Check sheet for the drawn part. Datum: minimum x, y, z corner. Units: mm. A direction names the side the tool comes from. Round coordinates to 2 decimals unless told otherwise and drop trailing zeros. Put each result on its own line as item: value.
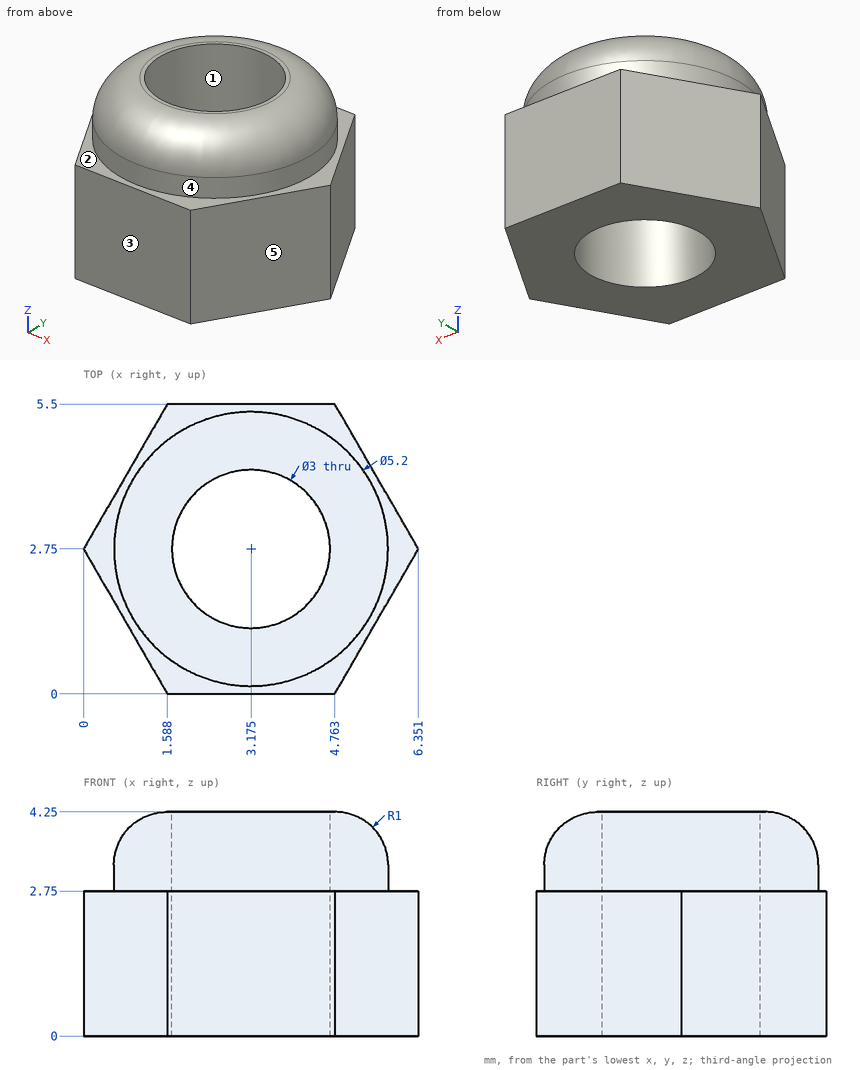
1. Access from +Z, -Z, +X, -X, +Y, -Y to the whole of each face (thin tool, end or side, straight path). Record for the marked faces 4 and 5.
Computed values:
face 4: +Z
face 5: +Z, -Z, +X, -Y
2. Release check for a two-part mould opening along Y. For the marked faces 1, 2 and 3 record: +Y half, -Y half, draft (parallel to the pull), parting line (faces both ways), or undercut.
Computed values:
face 1: undercut
face 2: draft
face 3: -Y half
3. Depth check by flat-ended pin: pin 1 Ø1 at (y, z) = (4, 0.5) entering from +X; pin 2 Ø1 at (x, z) = (1, 2) entering from -Y; pin 3 Ø2.5 at (x, y) = (3.18, 2.75) entering from -Z. Enter the tip coordinate at first touch or a pass-through.
Computed values:
pin 1: stops at x = 5.92
pin 2: stops at y = 0.15
pin 3: passes through
4. Scan lines: probe 1 along Y at (x, z) = (3.25, 1.45); probe 2 along Z at (x, y) = (6, 2.25); probe 3 along Y at (x, z) = (3.25, 2.95). Record each from-to range of solid material in increasing order.
Computed values:
probe 1: y = 0 to 1.25, 4.25 to 5.5
probe 2: z = 0 to 2.75
probe 3: y = 0.15 to 1.25, 4.25 to 5.35
